Could you check a few things on this model? Use its own coordinates, in mm. A direction names the side the tool comes from. Coordinates: 2 decimals unless noted, no trailing zeros. Write each loop counter-clockwise with the first axis right and the second up, starting at its lowest first coordinate (ties: lowest second). Pieces come first, ordered by that corner, then holes. Notation, with made-up numbers: M 33,46 L 58,46 A19 ccw 58,62 Z; hole C -26,55 d1. An arc over 180 degrees is marked long. Answer as CSV lines item,"result". Start each with the question number.
Item 1: I'm going to push flat-ended pins straight in: P1, Ø3, axis at x = 0.5, z = 2.5, coming from the +Y side; P2, Ø2, axis at x = 0.5, z = -6.5, coming from the -Y side. Where does each tip first touch, or does it pass through?
Item 2: Suppose I cut it at D-D, the plane y = 1.2. Write out the boundary of the cut face in (x, z), and give its area (3 significant figures).
Item 3: If I drill on line 1 along X through (y, z) = (0, 4.25); line 2 along Y through (x, z) = (0, -4.5); line 3 along Y through (x, z) = (1.2, 2.25), over which ranges is the centre line in solid material (lowest first)? Write a range as [from, to].
Item 4: Suppose I cut it at C-C, the plane x = 1.35. Write out the boundary of the cut face in (y, z).
Item 5: Suppose I cut it at B-B, the plane x = 0.2. Write out the boundary of the cut face in (y, z).
Item 6: We'd pull the mould along Y, two halves only. Please class faces 1 (the cylindrical face through (0.587, -0.747, -0.373)), 2 (the flat face through (0, -2.2, -0.5)), 3 (the flat face through (0, 1.85, 4)): +Y half, -Y half, draft (parallel to the pull), parting line (faces both ways), or undercut.
Item 7: On a 3-axis mill with a long thin cutter (end or side, diameter ignored), from which of +Z, -Z, +X, -X, +Y, -Y can I reach the whole of each face in a straight line? I mean faces 4 (the flat face through (0, 2.2, 0)), 5 (the flat face through (0, 2.2, -0.5)), 6 (the flat face through (-1, 1, -9)), 7 (the flat face through (0, -2.2, 0)), 8 (the flat face through (0, -1.85, -5)). Say none if no direction works.
Item 8: Suppose I cut it at A-A, the plane z = -2.75. Write out the boundary of the cut face in (x, y), and give its area (3 significant figures).
```python
from build123d import *

# Parameters (mm, degrees)
BOSS_EXTRUDE2_DEPTH = 8.5
BOSS_EXTRUDE4_START = 9
SKETCH3_R           = 2.700000061
SKETCH3_R_2         = 0.950000005
BOSS_EXTRUDE4_DEPTH = 9
SKETCH4_R           = 0.950000005
CUT_EXTRUDE1_DEPTH  = 8.5


with BuildPart() as part:
    # Sketch2 → Boss-Extrude2 (new body)
    with BuildSketch(Plane.XY):
        with BuildLine():
            Line((0, 0.950000005), (0, 1.85))
            Line((0, 1.85), (-1.966596128, 1.85))
            ThreePointArc((-1.966596128, 1.85), (-2.700000061, 0), (-1.966596128, -1.85))
            Line((-1.966596128, -1.85), (0, -1.85))
            Line((0, -1.85), (0, -0.950000005))
            ThreePointArc((0, -0.950000005), (-0.950000005, 0), (0, 0.950000005))
        make_face()
        with BuildLine():
            Line((1.966596128, 1.85), (0, 1.85))
            Line((0, 1.85), (0, 0.950000005))
            ThreePointArc((0, 0.950000005), (0.671751446, 0.671751446), (0.950000005, 0))
            ThreePointArc((0.950000005, 0), (0.671751446, -0.671751446), (0, -0.950000005))
            Line((0, -0.950000005), (0, -1.85))
            Line((0, -1.85), (1.966596128, -1.85))
            ThreePointArc((1.966596128, -1.85), (2.700000061, 0), (1.966596128, 1.85))
        make_face()
    extrude(amount=BOSS_EXTRUDE2_DEPTH)

    # Sketch3 → Boss-Extrude4 (add)
    with BuildSketch(Plane(origin=(0, 0, 0), x_dir=(-1, 0, 0), z_dir=(0, 0, -1)).offset(BOSS_EXTRUDE4_START)):
        Circle(SKETCH3_R)
        Circle(SKETCH3_R_2, mode=Mode.SUBTRACT)
    extrude(amount=-BOSS_EXTRUDE4_DEPTH)

    # Sketch4 → Cut-Extrude1 (cut)
    with BuildSketch(Plane(origin=(0, 0, -9), x_dir=(-1, 0, 0), z_dir=(0, 0, -1))):
        Circle(SKETCH4_R)
        with BuildLine():
            Line((-1.966596128, 1.85), (1.966596128, 1.85))
            ThreePointArc((1.966596128, 1.85), (0, 2.700000061), (-1.966596128, 1.85))
        make_face()
        with BuildLine():
            Line((1.966596128, -1.85), (-1.966596128, -1.85))
            ThreePointArc((-1.966596128, -1.85), (0, -2.700000061), (1.966596128, -1.85))
        make_face()
    extrude(amount=-CUT_EXTRUDE1_DEPTH, mode=Mode.SUBTRACT)


solid = part.part
```
Ans:
1,P1,"stops at y = 1.85"
1,P2,"stops at y = -1.85"
2,outline,"M -2.42,-9 L 2.42,-9 L 2.42,8.5 L -2.42,8.5 Z"
2,area,"84.7 mm^2"
3,line 1,"x = [-2.7, -0.95], [0.95, 2.7]"
3,line 2,"y = [-1.85, -0.95], [0.95, 1.85]"
3,line 3,"y = [-1.85, 1.85]"
4,outline,"M -2.34,-0.5 L -1.85,-0.5 L -1.85,-9 L 1.85,-9 L 1.85,-0.5 L 2.34,-0.5 L 2.34,0 L 1.85,0 L 1.85,8.5 L -1.85,8.5 L -1.85,0 L -2.34,0 Z"
5,outline,"M -2.69,-0.5 L -1.85,-0.5 L -1.85,-9 L -0.93,-9 L -0.93,8.5 L -1.85,8.5 L -1.85,0 L -2.69,0 Z; M 0.93,-9 L 1.85,-9 L 1.85,-0.5 L 2.69,-0.5 L 2.69,0 L 1.85,0 L 1.85,8.5 L 0.93,8.5 Z"
6,face 1,"undercut"
6,face 2,"draft"
6,face 3,"+Y half"
7,face 4,"+Z, +X, -X, +Y"
7,face 5,"-Z, +X, -X, +Y"
7,face 6,"-Z, +X, -X, +Y, -Y"
7,face 7,"+Z, +X, -X, -Y"
7,face 8,"-Z, +X, -X, -Y"
8,outline,"M -1.97,-1.85 L 1.97,-1.85 A2.7 ccw 1.97,1.85 L -1.97,1.85 A2.7 ccw Z; hole C 0,0 d1.9"
8,area,"15.4 mm^2"
